Source: CAD feature listing. Evaluate the final solid. Frame: model axes, mm. A direction names the side the tool comes from. Coordinates: 2 decimals unless noted, no trailing zeros. Write each loop counter-clockwise with the first axis right and the second up, starting at its lowest first coordinate (ties: lowest second). Pieces come first, ordered by that corner, then holes. Notation, with made-up numbers: (25, 77) - (44, 77) arc R18 cw to (44, 108) - close; hole circle Ø9 at (-26, 24). An arc over 180 degrees is marked (long way). One line per question, with ' | ' between items. Start each with the question number.
Q1. Cut plane B-B, the plane z = 20. Return loops of the section in (x, y), plus the area to 3 significant figures.
Q2. Draft query along Z for faces 1 (the face through (54, 2, 59)), 2 (the face through (28, 2, 56.976)), 3 (the face through (0, 2, 9.476)), 4 (the face through (0, 2, -26.524)). Return one class per face: +Z half, -Z half, draft (parallel to the pull), parting line (faces both ways), or undercut.
Q3. Contact query for flat-ended pins moving along their axis: P1, Ø2, axis at y = 2, z = 3, coming from the -X side; P2, Ø1.5, axis at y = 3, z = 26.5, coming from the +X side; P3, Ø1.5, axis at x = 48, y = 3.5, coming from the +Z side. Output: stop coordinate, or through.
Q4. Access query for faces 5 (the face through (30, 2, 59)), 6 (the face through (-14, 2, -36)), 7 (the face through (-54, 2, 59)), 8 (the face through (2, 2, 12)). Directions: +Z, -Z, +X, -X, +Y, -Y. A direction counts if a zero-diameter tool reaches every point of the face in a straight line with its end or side. Return the directions, or none.
Q5. Cut plane C-C, the plane y = 2.6. Give the number of separate pieces and of enclosed holes in the cut face, plus the area to 3 significant figures.
Q6. Cut plane D-D, the plane x = 20. Return loops of the section in (y, z).
Q7. Line query: line 1 (X direction, y = 3, z = 46); line 2 (Z direction, x = -57.5, y = 3.1); line 3 (X direction, y = 0.8, z = -29). Output: solid intervals per line, ascending.
Q8. Cut plane A-A, the plane z = -20. Return loops of the section in (x, y), plus the area to 3 significant figures.
```python
from build123d import *

# Parameters (mm, degrees)
SKETCH1_W           = 4
SKETCH1_H           = 4
BOSS_EXTRUDE1_DEPTH = 4
SKETCH2_W           = 4
SKETCH2_H           = 4
BOSS_EXTRUDE2_DEPTH = 4
CUT_EXTRUDE2_DEPTH  = 4


with BuildPart() as part:
    # Sketch1 → Boss-Extrude1 (new body)
    with BuildSketch(Plane(origin=(0, 0, 0), x_dir=(1, 0, 0), z_dir=(0, 1, 0))):
        Polygon((-66, 34.024336283), (-2, 34.024336283), (-2, 26.524336283), (2, 26.524336283), (2, 34.024336283), (66, 34.024336283), (58, -56.975663717), (2, -56.975663717), (2, -49.475663717), (-2, -49.475663717), (-2, -56.975663717), (-58, -56.975663717), align=None)
        with Locations((0, -3.475663717)):
            Rectangle(SKETCH1_W, SKETCH1_H, mode=Mode.SUBTRACT)
        with Locations((0, -11.475663717)):
            Rectangle(SKETCH1_W, SKETCH1_H, mode=Mode.SUBTRACT)
        with Locations((0, 4.524336283)):
            Rectangle(SKETCH1_W, SKETCH1_H, mode=Mode.SUBTRACT)
        with Locations((0, 12.524336283)):
            Rectangle(SKETCH1_W, SKETCH1_H, mode=Mode.SUBTRACT)
        with Locations((0, 20.524336283)):
            Rectangle(SKETCH1_W, SKETCH1_H, mode=Mode.SUBTRACT)
        with Locations((0, -19.475663717)):
            Rectangle(SKETCH1_W, SKETCH1_H, mode=Mode.SUBTRACT)
        with Locations((0, -27.475663717)):
            Rectangle(SKETCH1_W, SKETCH1_H, mode=Mode.SUBTRACT)
        with Locations((0, -35.475663717)):
            Rectangle(SKETCH1_W, SKETCH1_H, mode=Mode.SUBTRACT)
        with Locations((0, -43.475663717)):
            Rectangle(SKETCH1_W, SKETCH1_H, mode=Mode.SUBTRACT)
    extrude(amount=BOSS_EXTRUDE1_DEPTH)

    # Sketch2 → Boss-Extrude2 (add)
    with BuildSketch(Plane(origin=(0, 4, 0), x_dir=(1, 0, 0), z_dir=(0, 1, 0))):
        with Locations((-8, 36.024336283)):
            Rectangle(SKETCH2_W, SKETCH2_H)
        with Locations((-16, 36.024336283)):
            Rectangle(SKETCH2_W, SKETCH2_H)
        with Locations((-24, 36.024336283)):
            Rectangle(SKETCH2_W, SKETCH2_H)
        with Locations((-32, 36.024336283)):
            Rectangle(SKETCH2_W, SKETCH2_H)
        with Locations((56, 36.024336283)):
            Rectangle(SKETCH2_W, SKETCH2_H)
        with Locations((32, 36.024336283)):
            Rectangle(SKETCH2_W, SKETCH2_H)
        with Locations((-56, 36.024336283)):
            Rectangle(SKETCH2_W, SKETCH2_H)
        with Locations((24, 36.024336283)):
            Rectangle(SKETCH2_W, SKETCH2_H)
        with Locations((16, 36.024336283)):
            Rectangle(SKETCH2_W, SKETCH2_H)
        with Locations((8, 36.024336283)):
            Rectangle(SKETCH2_W, SKETCH2_H)
        with Locations((8, -58.975663717)):
            Rectangle(SKETCH2_W, SKETCH2_H)
        with Locations((16, -58.975663717)):
            Rectangle(SKETCH2_W, SKETCH2_H)
        with Locations((24, -58.975663717)):
            Rectangle(SKETCH2_W, SKETCH2_H)
        with Locations((32, -58.975663717)):
            Rectangle(SKETCH2_W, SKETCH2_H)
        with Locations((-52, -58.975663717)):
            Rectangle(SKETCH2_W, SKETCH2_H)
        with Locations((52, -58.975663717)):
            Rectangle(SKETCH2_W, SKETCH2_H)
        with Locations((-32, -58.975663717)):
            Rectangle(SKETCH2_W, SKETCH2_H)
        with Locations((-24, -58.975663717)):
            Rectangle(SKETCH2_W, SKETCH2_H)
        with Locations((-16, -58.975663717)):
            Rectangle(SKETCH2_W, SKETCH2_H)
        with Locations((-8, -58.975663717)):
            Rectangle(SKETCH2_W, SKETCH2_H)
    extrude(amount=-BOSS_EXTRUDE2_DEPTH)

    # Sketch3 → Cut-Extrude2 (cut)
    with BuildSketch(Plane(origin=(0, 4, 0), x_dir=(1, 0, 0), z_dir=(0, 1, 0))):
        with BuildLine():
            Line((-54, 34.024336283), (-54, 16.024336283))
            ThreePointArc((-54, 16.024336283), (-53.414213562, 14.610122721), (-52, 14.024336283))
            Line((-52, 14.024336283), (-36, 14.024336283))
            ThreePointArc((-36, 14.024336283), (-34.585786438, 14.610122721), (-34, 16.024336283))
            Line((-34, 16.024336283), (-34, 34.024336283))
            Line((-34, 34.024336283), (-54, 34.024336283))
        make_face()
        with BuildLine():
            Line((54, 34.024336283), (34, 34.024336283))
            Line((34, 34.024336283), (34, 16.024336283))
            ThreePointArc((34, 16.024336283), (34.585786438, 14.610122721), (36, 14.024336283))
            Line((36, 14.024336283), (52, 14.024336283))
            ThreePointArc((52, 14.024336283), (53.414213562, 14.610122721), (54, 16.024336283))
            Line((54, 16.024336283), (54, 34.024336283))
        make_face()
        with BuildLine():
            Line((-34, -56.975663717), (-50, -56.975663717))
            Line((-50, -56.975663717), (-50, -38.975663717))
            ThreePointArc((-50, -38.975663717), (-49.414213562, -37.561450154), (-48, -36.975663717))
            Line((-48, -36.975663717), (-36, -36.975663717))
            ThreePointArc((-36, -36.975663717), (-34.585786438, -37.561450154), (-34, -38.975663717))
            Line((-34, -38.975663717), (-34, -56.975663717))
        make_face()
        with BuildLine():
            Line((34, -56.975663717), (50, -56.975663717))
            Line((50, -56.975663717), (50, -38.975663717))
            ThreePointArc((50, -38.975663717), (49.414213562, -37.561450154), (48, -36.975663717))
            Line((48, -36.975663717), (36, -36.975663717))
            ThreePointArc((36, -36.975663717), (34.585786438, -37.561450154), (34, -38.975663717))
            Line((34, -38.975663717), (34, -56.975663717))
        make_face()
    extrude(amount=-CUT_EXTRUDE2_DEPTH, mode=Mode.SUBTRACT)


solid = part.part
```
Reply:
1) outline: (-61.25, 0) - (-2, 0) - (-2, 4) - (-61.25, 4) - close; (2, 0) - (61.25, 0) - (61.25, 4) - (2, 4) - close | area: 474 mm^2
2) face 1: draft | face 2: +Z half | face 3: undercut | face 4: -Z half
3) P1: stops at x = -62.83 | P2: stops at x = 60.75 | P3: stops at z = 37.12
4) face 5: +Z, +Y, -Y | face 6: -Z, +Y, -Y | face 7: +Z, -X, +Y, -Y | face 8: +Y, -Y
5) separate pieces: 1 | enclosed holes: 9 | area: 9,970 mm^2
6) outline: (0, -34.02) - (4, -34.02) - (4, 56.98) - (0, 56.98) - close
7) line 1: x = -58.96 to -50, -34 to 34, 50 to 58.96 | line 2: z = -38.02 to 56.98 | line 3: x = -65.56 to -54, -34 to -2, 2 to 34, 54 to 65.56
8) outline: (-64.77, 0) - (-54, 0) - (-54, 4) - (-64.77, 4) - close; (-34, 0) - (-2, 0) - (-2, 4) - (-34, 4) - close; (2, 0) - (34, 0) - (34, 4) - (2, 4) - close; (54, 0) - (64.77, 0) - (64.77, 4) - (54, 4) - close | area: 342 mm^2
